Check sheet for the modelled part. Datum: model origin and axes. Units: mm. A direction names the side the tool comes from. Give positions to 0.01 mm unless a question says otherwise; leave off trailing zeros. Order: outer loops, then holes, each group sorted by start corner. A loop starts at its lowest first (then second) coordinate and runs counter-clockwise, first axis right, second up.
```python
from build123d import *
from OCP.BRepFilletAPI import BRepFilletAPI_MakeChamfer

# Parameters (mm, degrees)
CUT_EXTRUDE2_REACH = 104.308
FILLET1_R          = 1
CIRPATTERN6_COUNT  = 5
CHAMFER2_SIZE      = 1
CHAMFER2_SIZE2     = 1.174957012


with BuildPart() as part:
    # Sketch1 → Revolve1 (revolve)
    with BuildSketch(Plane.XY, mode=Mode.PRIVATE) as revolve1_sk:
        Polygon((0, 12), (0, 25), (15, 25), (15, 61), (26, 61), (26, 27.183796727), (70, 21), (70, 16), (38, 16), (38, 8), (12, 8), (12, 12), align=None)
    revolve(revolve1_sk.sketch.rotate(Axis((0, 0, 0), (1, 0, 0)), 90), axis=Axis((0, 0, 0), (1, 0, 0)))

    # Sketch3 → Cut-Extrude2 (cut, up to next)
    with BuildSketch(Plane.ZY.offset(-15), mode=Mode.PRIVATE) as cut_extrude2_sk1:
        with BuildLine():
            Line((-11.877704642, 52.683141673), (-16.172703347, 58.817035512))
            ThreePointArc((-16.172703347, 58.817035512), (0, 61), (16.172703347, 58.817035512))
            Line((16.172703347, 58.817035512), (11.877704642, 52.683141673))
            ThreePointArc((11.877704642, 52.683141673), (0, 46.5), (-11.877704642, 52.683141673))
        make_face()
    cut_extrude2_tool1 = extrude(cut_extrude2_sk1.sketch, amount=-CUT_EXTRUDE2_REACH, mode=Mode.PRIVATE) & part.part
    cut_extrude2 = cut_extrude2_tool1.solids().sort_by_distance((15, 54.623829, 0))[0]
    add(cut_extrude2, mode=Mode.SUBTRACT)

    # Fillet1
    fillet1_edges = [part.edges().sort_by_distance(p)[0] for p in [
        (38, 0, -16),
        (26, 0, -27.183796727),
        (15, 0, -25),
        (12, 0, -12),
    ]]
    fillet(fillet1_edges, radius=FILLET1_R)

    # Sketch6 → M3 Clearance Hole2 (revolve, cut)
    with BuildSketch(Plane(origin=(15, 40.450849719, -29.389262615), x_dir=(0, 0, 1), z_dir=(0, 1, 0))):
        Polygon((0, 0), (0, 11), (4.525, 11), (4.5, 10.975), (4.5, 0.025), (4.525, 0), align=None)
    m3_clearance_hole2 = revolve(axis=Axis((8.65, 40.450849719, -29.389262615), (1, 0, 0)), mode=Mode.SUBTRACT)

    # CirPattern6: Cut-Extrude2, M3 Clearance Hole2 ×5 about axis
    cirpattern6_axis = Axis((0, 0, 0), (1, 0, 0))
    add([cut_extrude2.rotate(cirpattern6_axis, i * 360 / CIRPATTERN6_COUNT) for i in range(1, CIRPATTERN6_COUNT)], mode=Mode.SUBTRACT)
    add([m3_clearance_hole2.rotate(cirpattern6_axis, i * 360 / CIRPATTERN6_COUNT) for i in range(1, CIRPATTERN6_COUNT)], mode=Mode.SUBTRACT)

    # Chamfer2: one chamfer whose edges measure the first distance from different faces: ONE call of the kernel's chamfer builder (chamfer() names one face for all edges)
    chamfer2_edges_1 = [part.edges().sort_by_distance(p)[0] for p in [
        (26, 3.888963162, 57.355511424),
        (38, 0, -8),
        (26, 14.369290238, 44.224128008),
        (26, 30.566486464, 48.687458656),
        (15, 30.566486464, 48.687458656),
        (15, 14.369290238, 44.224128008),
        (15, 3.888963162, 57.355511424),
        (70, 0, -16),
        (0, 0, -25),
        (0, 0, -12),
        (26, 49.350036657, -35.85490039),
        (15, 49.350036657, -35.85490039),
        (15, 46.5, 0),
        (15, 55.750088593, 14.025203995),
        (15, 55.750088593, -14.025203995),
        (26, 46.5, 0),
        (26, 55.750088593, -14.025203995),
        (26, 55.750088593, 14.025203995),
        (26, -18.850036657, -58.014447494),
        (26, -61, 0),
        (26, -18.850036657, 58.014447494),
        (26, 49.350036657, 35.85490039),
        (15, -18.850036657, -58.014447494),
        (15, -61, 0),
        (15, -18.850036657, 58.014447494),
        (15, 49.350036657, 35.85490039),
        (26, 30.566486464, -48.687458656),
        (26, 14.369290238, -44.224128008),
        (26, 3.888963162, -57.355511424),
        (15, 3.888963162, -57.355511424),
        (15, 14.369290238, -44.224128008),
        (15, 30.566486464, -48.687458656),
        (26, -36.858961041, -44.11570827),
        (26, -37.619290238, -27.332014232),
        (26, -53.346577178, -21.422451507),
        (15, -53.346577178, -21.422451507),
        (15, -37.619290238, -27.332014232),
        (15, -36.858961041, -44.11570827),
        (12, 0, -8),
        (26, -53.346577178, 21.422451507),
        (26, -37.619290238, 27.332014232),
        (26, -36.858961041, 44.11570827),
        (15, -36.858961041, 44.11570827),
        (15, -37.619290238, 27.332014232),
        (15, -53.346577178, 21.422451507),
    ]]
    chamfer2_edges_2 = [part.edges().sort_by_distance(p)[0] for p in [
        (70, 0, -21),
    ]]
    chamfer2_side_2 = [part.faces().sort_by_distance(p)[0] for p in [
        (70, 0, -20.406030304),
    ]]
    chamfer2 = BRepFilletAPI_MakeChamfer(part.part.solid().wrapped)
    for e in chamfer2_edges_1:
        chamfer2.Add(CHAMFER2_SIZE, e.wrapped)
    for e in chamfer2_edges_2:
        chamfer2.Add(CHAMFER2_SIZE, CHAMFER2_SIZE2, e.wrapped, chamfer2_side_2[0].wrapped)  # the first distance lies on this face
    add(Compound.cast(chamfer2.Shape()), mode=Mode.REPLACE)


solid = part.part
```
(1) Thickness scan on L1, parallel to Y at x = 23.5, z = 0; L2, parallel to X at y = -7, z = -31; L3, parallel to Y at x = 16.5, z = -47.5. Record the ranges inside material, lowest first.
(2) Tool access check on faces 1 (the face through (15.507, 55.51, 14.459)), 2 (the face through (20.437, 55.793, 14.055)), 3 (the face through (25.51, 30.91, -48.31)). Record the directions out of +Z, -Z, +X, -X, +Y, -Y that give a thin tool (end or side, any length) a straight path to the whole face; none if there is none.
(3) Release check for a two-part mould opening along Y. For faces 4 (the face through (20.42, 44.44, -27.31)), 5 (the face through (0, 10, -10)), 6 (the face through (25.51, 55.5, -14.47)) record: released by +Y, released by -Y, zero draft, split by the parting line, or undercut.
(4) Sectioned sample at C-C (x = 58). Enter the section's corners in (y, z), plus the area to 3 significant figures.
(5) Sectioned sample at A-A (z = 0). Count the separate pieces of the cut face and the enclosed holes in it, plus the area to 3 significant figures.
(6) Sectioned sample at B-B (y = 30). Enter the section's corners in (x, z).
(7) Go/stop test with flat-tipped pins: P1, Ø17.5, axis at y = -0.5, z = -1.5, coming from the -X side; P2, Ø11.5, axis at y = -15.45, z = -47.55, coming from the +X side; P3, Ø5.5, axis at y = 40.45, z = 29.39, coming from the +X side; P4, Ø1, axis at x = 51, y = -9, coming from the -Z side. Record where each tip stops, or that it passes through.
(8) Sectioned sample at D-D (x = 32). Enter the section's corners in (y, z), plus the area to 3 significant figures.
Values follow:
1. L1: y = -61 to -54.5, -45.5 to -8, 8 to 46.5
1. L2: x = 15 to 26
1. L3: y = -38.02 to -19.95, -10.95 to 8.87, 28.99 to 38.27
2. face 1: -X, +Y
2. face 2: +X, -X, +Y
2. face 3: -Z, +X
3. face 4: undercut
3. face 5: zero draft
3. face 6: released by +Y
4. outline: circle Ø45.37 at (0, 0); hole circle Ø32 at (0, 0)
4. area: 813 mm2
5. separate pieces: 3
5. enclosed holes: 0
5. area: 2,220 mm2
6. outline: (15, -47.01) - (16, -48.26) - (25, -48.26) - (26, -47.01) - (26, 47.01) - (25, 48.26) - (16, 48.26) - (15, 47.01) - close
7. P1: stops at x = 12
7. P2: stops at x = 26
7. P3: passes through
7. P4: stops at z = -22.11
8. outline: circle Ø52.68 at (0, 0); hole circle Ø16 at (0, 0)
8. area: 1,980 mm2
